from build123d import *

# Parameters (mm, degrees)
BOSS_EXTRUDE1_DEPTH      = 25.4
BOSS_EXTRUDE1_DEPTH_BACK = 25.4
SKETCH1_W                = 204.950025332
SKETCH1_H                = 72.158698858
SKETCH2_W                = 220.605080335
SKETCH2_H                = 76.557810487
SKETCH2_W_2              = 204.950025332
SKETCH2_H_2              = 50.8
SKETCH2_R                = 4.7625
CUT_EXTRUDE1_DEPTH       = 219.761401313
FILLET1_R                = 1.5875
CUT_EXTRUDE2_DEPTH       = 6.35
SKETCH4_R                = 1.5875
CUT_EXTRUDE3_DEPTH       = 12.7
SKETCH5_R                = 1.5875
CUT_EXTRUDE4_DEPTH       = 12.7


with BuildPart() as part:
    # Sketch1 → Boss-Extrude1 (new, two sides: drawn at the far end of the back side and taken through both)
    with BuildSketch(Plane.XY.offset(-BOSS_EXTRUDE1_DEPTH_BACK)):
        with Locations((102.475012666, 366.768835108)):
            Rectangle(SKETCH1_W, SKETCH1_H)
    extrude(amount=BOSS_EXTRUDE1_DEPTH + BOSS_EXTRUDE1_DEPTH_BACK)

    # Sketch2 → Cut-Extrude1 (cut, through all)
    # profile 1 of 6: a face of its own
    with BuildSketch(Plane(origin=(0, 402.848184537, 0), x_dir=(1, 0, 0), z_dir=(0, 1, 0))):
        with Locations((101.602425497, 0.332919425)):
            Rectangle(SKETCH2_W, SKETCH2_H)
        with Locations((102.475012666, 0)):
            Rectangle(SKETCH2_W_2, SKETCH2_H_2, mode=Mode.SUBTRACT)
    # profile 2 of 6: a face of its own
    with BuildSketch(Plane(origin=(0, 402.848184537, 0), x_dir=(1, 0, 0), z_dir=(0, 1, 0))):
        with BuildLine():
            Line((0, 25.4), (0, 0.179710991))
            ThreePointArc((0, 0.179710991), (0.318408098, 1.411023063), (1.193802692, 2.333626683))
            Line((1.193802692, 2.333626683), (36.555662769, 24.43478923))
            ThreePointArc((36.555662769, 24.43478923), (38.17057208, 25.153929538), (39.921156038, 25.4))
            Line((39.921156038, 25.4), (0, 25.4))
        make_face()
    # profile 3 of 6: a face of its own
    with BuildSketch(Plane(origin=(0, 402.848184537, 0), x_dir=(1, 0, 0), z_dir=(0, 1, 0))):
        with BuildLine():
            Line((36.555662769, -24.43478923), (1.193802692, -2.333626683))
            ThreePointArc((1.193802692, -2.333626683), (0.318408098, -1.411023063), (0, -0.179710991))
            Line((0, -0.179710991), (0, -25.4))
            Line((0, -25.4), (39.921156038, -25.4))
            ThreePointArc((39.921156038, -25.4), (38.17057208, -25.153929538), (36.555662769, -24.43478923))
        make_face()
    # profile 4 of 6: a face of its own
    with BuildSketch(Plane(origin=(0, 402.848184537, 0), x_dir=(1, 0, 0), z_dir=(0, 1, 0))):
        with BuildLine():
            ThreePointArc((168.394362563, -24.43478923), (166.779453252, -25.153929538), (165.028869294, -25.4))
            Line((165.028869294, -25.4), (204.950025332, -25.4))
            Line((204.950025332, -25.4), (204.950025332, -0.179710991))
            ThreePointArc((204.950025332, -0.179710991), (204.631617234, -1.411023063), (203.756222639, -2.333626683))
            Line((203.756222639, -2.333626683), (168.394362563, -24.43478923))
        make_face()
    # profile 5 of 6: a face of its own
    with BuildSketch(Plane(origin=(0, 402.848184537, 0), x_dir=(1, 0, 0), z_dir=(0, 1, 0))):
        with BuildLine():
            Line((204.950025332, 25.4), (165.028869294, 25.4))
            ThreePointArc((165.028869294, 25.4), (166.779453252, 25.153929538), (168.394362563, 24.43478923))
            Line((168.394362563, 24.43478923), (203.756222639, 2.333626683))
            ThreePointArc((203.756222639, 2.333626683), (204.631617234, 1.411023063), (204.950025332, 0.179710991))
            Line((204.950025332, 0.179710991), (204.950025332, 25.4))
        make_face()
    # profile 6 of 6: a face of its own
    with BuildSketch(Plane(origin=(0, 402.848184537, 0), x_dir=(1, 0, 0), z_dir=(0, 1, 0))):
        with Locations(Location((102.475012666, -0.179710991, 0), (0, 0, 270))):
            Circle(SKETCH2_R)
    extrude(amount=-CUT_EXTRUDE1_DEPTH, mode=Mode.SUBTRACT)

    # Fillet1
    fillet1_edges = [part.edges().sort_by_distance(p)[0] for p in [
        (102.475012666, 330.689485679, 25.4),
        (102.475012666, 402.848184537, 25.4),
        (102.475012666, 402.848184537, -25.4),
        (102.475012666, 330.689485679, -25.4),
        (204.950025332, 330.689485679, 0),
        (0, 330.689485679, 0),
        (204.950025332, 402.848184537, 0),
        (0, 402.848184537, 0),
        (204.631617234, 330.689485679, -1.411023063),
        (186.075292601, 330.689485679, -13.384207957),
        (166.779453252, 330.689485679, -25.153929538),
        (0.318408098, 330.689485679, -1.411023063),
        (38.17057208, 330.689485679, -25.153929538),
        (18.874732731, 330.689485679, -13.384207957),
        (204.631617234, 330.689485679, 1.411023063),
        (166.779453252, 330.689485679, 25.153929538),
        (186.075292601, 330.689485679, 13.384207957),
        (38.17057208, 402.848184537, -25.153929538),
        (18.874732731, 402.848184537, -13.384207957),
        (0.318408098, 402.848184537, -1.411023063),
        (0.318408098, 330.689485679, 1.411023063),
        (18.874732731, 402.848184537, 13.384207957),
        (38.17057208, 402.848184537, 25.153929538),
        (166.779453252, 402.848184537, 25.153929538),
        (186.075292601, 402.848184537, 13.384207957),
        (204.631617234, 402.848184537, 1.411023063),
        (204.631617234, 402.848184537, -1.411023063),
        (186.075292601, 402.848184537, -13.384207957),
        (166.779453252, 402.848184537, -25.153929538),
        (18.874732731, 330.689485679, 13.384207957),
        (38.17057208, 330.689485679, 25.153929538),
        (0.318408098, 402.848184537, 1.411023063),
    ]]
    fillet(fillet1_edges, radius=FILLET1_R)

    # Sketch3 → Cut-Extrude2 (cut)
    with BuildSketch(Plane.XY.offset(25.4)):
        with BuildLine():
            ThreePointArc((42.179379055, 360.341209381), (101.998613328, 386.003937421), (161.817847601, 360.341209381))
            ThreePointArc((161.817847601, 360.341209381), (162.494976111, 358.255146927), (161.294952196, 356.419363121))
            ThreePointArc((161.294952196, 356.419363121), (101.998613328, 339.835452874), (42.702274459, 356.419363121))
            ThreePointArc((42.702274459, 356.419363121), (41.502250545, 358.255146927), (42.179379055, 360.341209381))
        make_face()
    cut_extrude2 = extrude(amount=-CUT_EXTRUDE2_DEPTH, mode=Mode.SUBTRACT)

    # Mirror1: Cut-Extrude2 across plane
    add(cut_extrude2.mirror(Plane.XY), mode=Mode.SUBTRACT)

    # Sketch4 → Cut-Extrude3 (cut)
    with BuildSketch(Plane.XZ.offset(-330.689485679)):
        with Locations(Location((92.950012666, 0.179710991, 0), (0, 0, 270))):
            Circle(SKETCH4_R)
        with Locations(Location((112.000012666, 0.179710991, 0), (0, 0, 270))):
            Circle(SKETCH4_R)
    extrude(amount=-CUT_EXTRUDE3_DEPTH, mode=Mode.SUBTRACT)

    # Sketch5 → Cut-Extrude4 (cut)
    with BuildSketch(Plane(origin=(0, 402.848184537, 0), x_dir=(1, 0, 0), z_dir=(0, 1, 0))):
        with Locations(Location((89.775012666, -0.179710991, 0), (0, 0, 270))):
            Circle(SKETCH5_R)
        with Locations(Location((115.175012666, -0.179710991, 0), (0, 0, 270))):
            Circle(SKETCH5_R)
    extrude(amount=-CUT_EXTRUDE4_DEPTH, mode=Mode.SUBTRACT)


solid = part.part
Geometry check sheet. Reference: the model listing, model coordinates, mm. A direction names the side the tool comes from. Give positions to 0.01 mm unless a question says otherwise; leave off trailing zeros. Answer as a JSON object with one key per item and string values. Group by question number.
Item 1: Sectioned sample at B-B on y = 392. Give the number of separate pieces and of enclosed holes in the cut face, plus the area to 3 significant figures.
Item 2: Gauge pin test, flat ends, axial feed: pin 1 (1 mm diameter, centred on x = 115.5, z = 0, fed in from +Y); pin 2 (1 mm diameter, centred on y = 377, z = 5, fed in from -X); pin 3 (6 mm diameter, centred on y = 384.5, z = 14, fed in from +X). Record the tip position at first contact, or that the pin passes through.
Item 3: Access from +Z, -Z, +X, -X, +Y, -Y to the whole of each face (thin tool, end or side, straight path). Record for faces 1 (the flat face through (103, 363, -19.05)), 2 (the cylindrical face through (101.1, 386, 22.3)), 3 (the flat face through (101, 402.848, 5)).
Item 4: Mould release check, pull along X, two halves, no side actions. Record for faces 4 (the cylindrical face through (41.507, 358.224, 22.269)), 5 (the flat face through (186.32, 367.25, 13.23)), 6 (the cylindrical face through (19.4, 331.1, 13.1)): pulls with the +X half, pulls with the -X half, needs draft (parallel to the pull), parting line crosses it, or undercut.
Item 5: Material ranges on L1, parallel to X at y = 400.5, z = -1; L2, parallel to X at y = 393, z = -0.5; L3, parallel to Y at x = 100, z = 22, recorded low to high.
Findings below:
{
 "1": {"separate pieces": "1", "enclosed holes": "3", "area": "8,510 mm2"},
 "2": {"pin 1": "y = 390.15", "pin 2": "x = 4.66", "pin 3": "x = 189.89"},
 "3": {"face 1": "-Z", "face 2": "+Z", "face 3": "+Z, -Z, +X, -X, +Y"},
 "4": {"face 4": "undercut", "face 5": "pulls with the +X half", "face 6": "pulls with the -X half"},
 "5": {"L1": "0.14 to 88.71, 90.84 to 97.86, 107.09 to 114.11, 116.24 to 204.81", "L2": "0.02 to 88.34, 91.21 to 97.76, 107.19 to 113.74, 116.61 to 204.93", "L3": "330.69 to 339.85, 385.98 to 402.85"}
}
